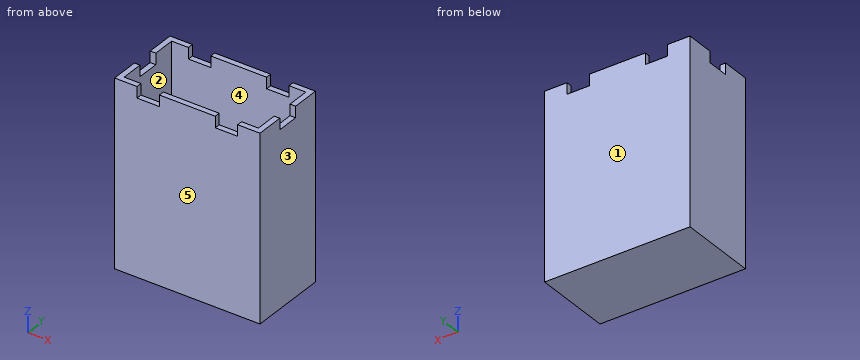
```python
from build123d import *

# Parameters (mm, degrees)
F0_W     = 130
F0_H     = 70
F1_DEPTH = 5
F2_W     = 130
F2_H     = 70
F2_W_2   = 120
F2_H_2   = 60
F3_DEPTH = 160
F4_W     = 20
F4_H     = 25
F4_H_2   = 20
F4_W_2   = 50
F5_DEPTH = 10


with BuildPart() as f1:
    # F0 (on Top) → F1 (new body)
    with BuildSketch(Plane.XY):
        with Locations((65, 35)):
            Rectangle(F0_W, F0_H)
    extrude(amount=F1_DEPTH)

    # F2 (on face) → F3 (join)
    with BuildSketch(Plane.XY.offset(5)):
        with Locations((65, 35)):
            Rectangle(F2_W, F2_H)
        with Locations((65, 35)):
            Rectangle(F2_W_2, F2_H_2, mode=Mode.SUBTRACT)
    extrude(amount=F3_DEPTH)

    # F4 (on face) → F5 (cut)
    with BuildSketch(Plane.XY.offset(165)):
        with Locations((30, 12.5)):
            Rectangle(F4_W, F4_H)
        with Locations((10, 35)):
            Rectangle(F4_W, F4_H_2)
        with Locations((65, 35)):
            Rectangle(F4_W_2, F4_H_2)
        with Locations((30, 57.5)):
            Rectangle(F4_W, F4_H)
        with Locations((100, 12.5)):
            Rectangle(F4_W, F4_H)
        with Locations((100, 57.5)):
            Rectangle(F4_W, F4_H)
        with Locations((120, 35)):
            Rectangle(F4_W, F4_H_2)
    extrude(amount=-F5_DEPTH, mode=Mode.SUBTRACT)


solid = f1.part
```
Build history of the part. All positions in model axes, mm. Face numbers are marked on the shaded views. A direction names the side the tool comes from. Give positions to 0.01 mm unless a question says otherwise; leave off trailing zeros. Loops run counter-clockwise (first coordinate to the right, second up) from the corner with the lowest first, then second, coordinate; pieces in that order, holes last. Notation, with made-up numbers: (-12.5, 21.5) - (41.5, 21.5) arc R6 cw to (41.5, 30.5) - close; hole circle Ø10 at (50.25, -29). An arc over 180 degrees is marked (long way). Use a Markdown table: item, result.
(1) Wall check: line 1 along Y through (x, z) = (86, 140.5); line 2 along X through (y, z) = (51, 81); line 3 along Z through (x, y) = (118.5, 47). Give the ranges that are in metal, low to high.
Taken from the geometry:
| item | result |
|---|---|
| line 1 | 0 to 5, 65 to 70 |
| line 2 | 0 to 5, 125 to 130 |
| line 3 | 0 to 5 |
(2) Which spindle directions (+Z, -Z, +X, -X, +Y, -Y) get a long thin tool onto all of the face, cutting with end or side? Do the marked faces 1 and 2. Say none if no direction does.
Taken from the geometry:
| item | result |
|---|---|
| face 1 | +Z, -Z, +X, -X, +Y |
| face 2 | +Z |
(3) Drop flat-ended pins along their axis: pin 1 Ø4 at (x, y) = (103, 2) entering from +Z; pin 2 Ø18 at (x, y) = (48, 24) entering from +Z. Give the stop position or say it passes through.
Taken from the geometry:
| item | result |
|---|---|
| pin 1 | z = 155 |
| pin 2 | z = 5 |
(4) Band-saw the part on C-C (x = 95.5). Give the cut face in (y, z), and give its area (3 significant figures).
Taken from the geometry:
| item | result |
|---|---|
| outline | (0, 0) - (70, 0) - (70, 155) - (65, 155) - (65, 5) - (5, 5) - (5, 155) - (0, 155) - close |
| area | 1,850 mm2 |
(5) Pull direction Y, two halves, no side cores. Call the marked faces 3, 4 and 5: +Y half, -Y half, draft (parallel to the pull), parting line (faces both ways), or undercut.
Taken from the geometry:
| item | result |
|---|---|
| face 3 | draft |
| face 4 | undercut |
| face 5 | -Y half |
(6) Band-saw the part on A-A (z = 20). Give the cut face in (x, y).
Taken from the geometry:
| item | result |
|---|---|
| outline | (0, 0) - (130, 0) - (130, 70) - (0, 70) - close; hole (5, 5) - (125, 5) - (125, 65) - (5, 65) - close |
(7) Band-saw the part on B-B (y = 29.5). Give the cut face in (x, z).
Taken from the geometry:
| item | result |
|---|---|
| outline | (0, 0) - (130, 0) - (130, 155) - (125, 155) - (125, 5) - (5, 5) - (5, 155) - (0, 155) - close |
